```python
from build123d import *

# Parameters (mm, degrees)
SKETCH1_R               = 2.0701
BOSS_EXTRUDE1_DEPTH     = 2.286
SKETCH2_W               = 25.273
SKETCH2_H               = 25.4
CUT_EXTRUDE1_DEPTH      = 1
CUT_EXTRUDE1_DEPTH_BACK = 3.286


with BuildPart() as part:
    # Sketch1 → Boss-Extrude1 (new body)
    with BuildSketch(Plane(origin=(0, 0, 0), x_dir=(-1, 0, 0), z_dir=(0, 0, -1))):
        with BuildLine():
            Line((10.414, 12.573), (-54.864, 12.573))
            Line((-54.864, 12.573), (-57.023, 10.414))
            Line((-57.023, 10.414), (-57.023, -10.668))
            Line((-57.023, -10.668), (-54.864, -12.827))
            Line((-54.864, -12.827), (-19.177, -12.827))
            ThreePointArc((-19.177, -12.827), (-14.686871939, -14.686871939), (-12.827, -19.177))
            Line((-12.827, -19.177), (-12.827, -54.864))
            Line((-12.827, -54.864), (-10.668, -57.023))
            Line((-10.668, -57.023), (10.414, -57.023))
            Line((10.414, -57.023), (12.573, -54.864))
            Line((12.573, -54.864), (12.573, 10.414))
            Line((12.573, 10.414), (10.414, 12.573))
        make_face()
        with Locations((0, -50.8)):
            Circle(SKETCH1_R, mode=Mode.SUBTRACT)
        with Locations((0, -25.4)):
            Circle(SKETCH1_R, mode=Mode.SUBTRACT)
        with Locations((-38.1, 0)):
            Circle(SKETCH1_R, mode=Mode.SUBTRACT)
        with Locations((-12.7, 0)):
            Circle(SKETCH1_R, mode=Mode.SUBTRACT)
        Circle(SKETCH1_R, mode=Mode.SUBTRACT)
        with Locations((-25.4, 0)):
            Circle(SKETCH1_R, mode=Mode.SUBTRACT)
        with Locations((0, -12.7)):
            Circle(SKETCH1_R, mode=Mode.SUBTRACT)
        with Locations((0, -38.1)):
            Circle(SKETCH1_R, mode=Mode.SUBTRACT)
        with Locations((-50.8, 0)):
            Circle(SKETCH1_R, mode=Mode.SUBTRACT)
    extrude(amount=-BOSS_EXTRUDE1_DEPTH)

    # Sketch2 → Cut-Extrude1 (cut, two sides)
    with BuildSketch(Plane.XY.offset(2.286)) as cut_extrude1_sk:
        with Locations((44.3865, -0.127)):
            Rectangle(SKETCH2_W, SKETCH2_H)
    extrude(amount=CUT_EXTRUDE1_DEPTH, mode=Mode.SUBTRACT)
    extrude(cut_extrude1_sk.sketch, amount=-CUT_EXTRUDE1_DEPTH_BACK, mode=Mode.SUBTRACT)


solid = part.part
```
The model under review builds one solid part; all positions refer to its coordinate system, in mm. A direction names the side the tool comes from. Give positions to 0.01 mm unless a question says otherwise; leave off trailing zeros. Write each loop counter-clockwise with the first axis right and the second up, starting at its lowest first coordinate (ties: lowest second). Pieces come first, ordered by that corner, then holes.
(1) To check wall thickness, follow L1, parallel to Y at x = 0, z = 1.4; L2, parallel to Y at x = 1, z = 0.35; L3, parallel to X at y = -44, z = 1. State the ranges of each line that lie inside material, in increasing order.
(2) Consider section C-C, the plane x = 0. Give the boundary of the cut face in (y, z).
(3) Tool access review of faces 4 (the flat face through (5, -14, 2.286)), 5 (the flat face through (12.827, -37, 1)): name each direction out of +Z, -Z, +X, -X, +Y, -Y from which nothing blocks a thin tool from reaching the whole face with its end or side.
(4) Consider section D-D, the plane x = 13.5. Give the boundary of the cut face in (y, z).
(5) For P1, Ø5.5, axis at x = 0, y = -38.1, coming from the -Z side; P2, Ø0.7, axis at y = -29.5, z = 1, coming from the +X side, all flat-tipped, find the tip position at first contact; note any pin that passes through.
(6) Consider section B-B, the plane z = 1.05. Give the boundary of the cut face in (x, y), and give its area (3 significant figures).
(7) The part is to be moulded in two halves that separate along Y. For faces 1 (the flat face through (-11.509, 11.478, 1.127)), 2 (the flat face through (26, -12.827, 1)), 3 (the cylindrical face through (14.226, 1.399, 1.127)), say which applies: released by +Y, released by -Y, zero draft, split by the parting line, or undercut.
(8) Consider section A-A, the plane y = -25.4. Give the boundary of the cut face in (x, z), and give its area (3 significant figures).
Returned:
1. L1: y = -57.02 to -52.87, -48.73 to -40.17, -36.03 to -27.47, -23.33 to -14.77, -10.63 to -2.07, 2.07 to 12.57
1. L2: y = -57.02 to -52.61, -48.99 to -39.91, -36.29 to -27.21, -23.59 to -14.51, -10.89 to -1.81, 1.81 to 12.57
1. L3: x = -12.57 to 12.83
2. outline: (-57.02, 0) - (-52.87, 0) - (-52.87, 2.29) - (-57.02, 2.29) - close; (-48.73, 0) - (-40.17, 0) - (-40.17, 2.29) - (-48.73, 2.29) - close; (-36.03, 0) - (-27.47, 0) - (-27.47, 2.29) - (-36.03, 2.29) - close; (-23.33, 0) - (-14.77, 0) - (-14.77, 2.29) - (-23.33, 2.29) - close; (-10.63, 0) - (-2.07, 0) - (-2.07, 2.29) - (-10.63, 2.29) - close; (2.07, 0) - (12.57, 0) - (12.57, 2.29) - (2.07, 2.29) - close
3. face 4: +Z, +X, -X, +Y, -Y
3. face 5: +Z, -Z, +X, -Y
4. outline: (-16.33, 0) - (-1.91, 0) - (-1.91, 2.29) - (-16.33, 2.29) - close; (1.91, 0) - (12.57, 0) - (12.57, 2.29) - (1.91, 2.29) - close
5. P1: stops at z = 0
5. P2: stops at x = 12.83
6. outline: (-12.57, -54.86) - (-10.41, -57.02) - (10.67, -57.02) - (12.83, -54.86) - (12.83, -19.18) arc R6.35 cw to (19.18, -12.83) - (31.75, -12.83) - (31.75, 12.57) - (-10.41, 12.57) - (-12.57, 10.41) - close; hole circle Ø4.14 at (0, -50.8); hole circle Ø4.14 at (0, -38.1); hole circle Ø4.14 at (0, -25.4); hole circle Ø4.14 at (0, -12.7); hole circle Ø4.14 at (0, 0); hole circle Ø4.14 at (12.7, 0); hole circle Ø4.14 at (25.4, 0)
6. area: 2,160 mm2
7. face 1: released by +Y
7. face 2: released by -Y
7. face 3: undercut
8. outline: (-12.57, 0) - (-2.07, 0) - (-2.07, 2.29) - (-12.57, 2.29) - close; (2.07, 0) - (12.83, 0) - (12.83, 2.29) - (2.07, 2.29) - close
8. area: 48.6 mm2
